from build123d import *

# Parameters (mm, degrees)
F0_W     = 42
F0_H     = 42
F1_DEPTH = 9.5
F3_DEPTH = 16.57
F4_W     = 42
F4_H     = 42
F5_DEPTH = 7.6
F7_DEPTH = 3
F8_R     = 2.5
F9_DEPTH = 24
F10_SIZE = 2
F11_R    = 1


with BuildPart() as f1:
    # F0 (on Top) → F1 (new body)
    with BuildSketch(Plane.XY):
        Rectangle(F0_W, F0_H)
    extrude(amount=F1_DEPTH)

    # F2 (on face) → F3 (join)
    with BuildSketch(Plane.XY.offset(9.5)):
        with BuildLine():
            Line((-16, -21), (16, -21))
            ThreePointArc((16, -21), (19.5355339059, -19.5355339059), (21, -16))
            Line((21, -16), (21, 16))
            ThreePointArc((21, 16), (19.5355339059, 19.5355339059), (16, 21))
            Line((16, 21), (-16, 21))
            ThreePointArc((-16, 21), (-19.5355339059, 19.5355339059), (-21, 16))
            Line((-21, 16), (-21, -16))
            ThreePointArc((-21, -16), (-19.5355339059, -19.5355339059), (-16, -21))
        make_face()
    extrude(amount=F3_DEPTH)

    # F4 (on face) → F5 (join)
    with BuildSketch(Plane.XY.offset(26.07)):
        Rectangle(F4_W, F4_H)
    extrude(amount=F5_DEPTH)

    # F6 (on face) → F7 (cut)
    with BuildSketch(Plane.XY.offset(33.67)):
        with BuildLine():
            Line((15.5, -14), (15.5, -15.5))
            Line((15.5, -15.5), (14, -15.5))
            ThreePointArc((14, -15.5), (15.5, -17), (17, -15.5))
            ThreePointArc((17, -15.5), (16.5606601718, -14.4393398282), (15.5, -14))
        make_face()
        with BuildLine():
            Line((14, -15.5), (15.5, -15.5))
            Line((15.5, -15.5), (15.5, -14))
            ThreePointArc((15.5, -14), (14.4393398282, -14.4393398282), (14, -15.5))
        make_face()
        with BuildLine():
            Line((15.5, 14), (15.5, 15.5))
            Line((15.5, 15.5), (14, 15.5))
            ThreePointArc((14, 15.5), (14.4393398282, 14.4393398282), (15.5, 14))
        make_face()
        with BuildLine():
            Line((14, 15.5), (15.5, 15.5))
            Line((15.5, 15.5), (15.5, 14))
            ThreePointArc((15.5, 14), (16.5606601718, 14.4393398282), (17, 15.5))
            ThreePointArc((17, 15.5), (15.5, 17), (14, 15.5))
        make_face()
        with BuildLine():
            Line((-14, -15.5), (-15.5, -15.5))
            Line((-15.5, -15.5), (-15.5, -14))
            ThreePointArc((-15.5, -14), (-16.5606601718, -16.5606601718), (-14, -15.5))
        make_face()
        with BuildLine():
            Line((-15.5, -14), (-15.5, -15.5))
            Line((-15.5, -15.5), (-14, -15.5))
            ThreePointArc((-14, -15.5), (-14.4393398282, -14.4393398282), (-15.5, -14))
        make_face()
        with BuildLine():
            Line((-15.5, 15.5), (-14, 15.5))
            ThreePointArc((-14, 15.5), (-16.5606601718, 16.5606601718), (-15.5, 14))
            Line((-15.5, 14), (-15.5, 15.5))
        make_face()
        with BuildLine():
            ThreePointArc((-15.5, 14), (-14.4393398282, 14.4393398282), (-14, 15.5))
            Line((-14, 15.5), (-15.5, 15.5))
            Line((-15.5, 15.5), (-15.5, 14))
        make_face()
    extrude(amount=-F7_DEPTH, mode=Mode.SUBTRACT)

    # F8 (on face) → F9 (join)
    with BuildSketch(Plane.XY.offset(33.67)):
        Circle(F8_R)
    extrude(amount=F9_DEPTH)

    # F10
    f10_edges = [f1.edges().sort_by_distance(p)[0] for p in [
        (21, 21, 29.87),
        (21, 21, 4.75),
        (-21, 21, 29.87),
        (-21, 21, 4.75),
        (-21, -21, 29.87),
        (-21, -21, 4.75),
        (21, -21, 4.75),
        (21, -21, 29.87),
    ]]
    chamfer(f10_edges, length=F10_SIZE)

    # F11
    f11_edges = [f1.edges().sort_by_distance(p)[0] for p in [
        (0, 21, 33.67),
        (-20, 20, 33.67),
        (-21, 0, 33.67),
        (-20, -20, 33.67),
        (0, -21, 33.67),
        (20, -20, 33.67),
        (21, 0, 33.67),
        (20, 20, 33.67),
        (0, 21, 0),
        (21, 0, 0),
        (20, 20, 0),
        (-21, 0, 0),
        (-20, 20, 0),
        (0, -21, 0),
        (20, -20, 0),
        (-20, -20, 0),
    ]]
    fillet(f11_edges, radius=F11_R)


solid = f1.part
The model under review builds one solid part; all positions refer to its coordinate system, in mm. A direction names the side the tool comes from. Coordinates: 2 decimals unless noted, no trailing zeros. Loops run counter-clockwise (first coordinate to the right, second up) from the corner with the lowest first, then second, coordinate; pieces in that order, holes last. Notation, with made-up numbers: (50, 9.25) -> (93, 9.25) arc R26 cw to (93, 35.25) -> close; hole circle Ø9 at (8.25, 89). An arc over 180 degrees is marked (long way). Use a Markdown table: item, result. Add a question column.
1. Add section A-A on x = 0. Write out the cut boundary in (y, z).
2. To check wall thickness, follow line 1 (X direction, y = -15.5, z = 32.55); line 2 (X direction, y = -15, z = 32). State the ranges of each line that lie inside material, in increasing order.
3. Add section C-C on z = 51.5. Write out the cut boundary in (x, y).
4. Clearance check with flat-ended pins moving along their axes: pin 1 Ø5.5 at (x, y) = (-19, -19.5) entering from +Z; pin 2 Ø0.9 at (x, y) = (-15.5, 15.5) entering from +Z; pin 3 Ø2 at (y, z) = (-1, 40.5) entering from +X. State where each tip first meets the part, or that it passes through.
5. Add section B-B on y = -7.5. Write out the cut boundary in (x, z), plus the area to 3 significant figures.
6. Draft analysis for pull direction Y (two halves, no side actions). For faces 5 (the face through (-20, 20, 5)), 6 (the face through (15, 16, 30.67)), 7 (the face through (-20, -19, 18)), state which applies: pulls with the +Y half, pulls with the -Y half, needs draft (parallel to the pull), parting line crosses it, or undercut.
7. Machinability: for faces 1 (the face through (19.6, 19.8, 9.5)), 2 (the face through (-16, -15, 30.67)), 3 (the face through (-19, 20, 18)), 4 (the face through (-19.8, -19.6, 26.07)), which of the approach directions +Z, -Z, +X, -X, +Y, -Y give a long, thin tool a straight path to every point of the face, cutting with its end or side? Answer none if there is none.
Returned:
| question | item | result |
|---|---|---|
| 1 | outline | (-21, 1) arc R1 ccw to (-20, 0) -> (20, 0) arc R1 ccw to (21, 1) -> (21, 32.67) arc R1 ccw to (20, 33.67) -> (2.5, 33.67) -> (2.5, 57.67) -> (-2.5, 57.67) -> (-2.5, 33.67) -> (-20, 33.67) arc R1 ccw to (-21, 32.67) -> close |
| 2 | line 1 | x = -21 to -17, -14 to 14, 17 to 21 |
| 2 | line 2 | x = -21 to -16.91, -14.09 to 14.09, 16.91 to 21 |
| 3 | outline | circle Ø5 at (0, 0) |
| 4 | pin 1 | stops at z = 33.67 |
| 4 | pin 2 | stops at z = 30.67 |
| 4 | pin 3 | stops at x = 2.5 |
| 5 | outline | (-21, 1) arc R1 ccw to (-20, 0) -> (20, 0) arc R1 ccw to (21, 1) -> (21, 32.67) arc R1 ccw to (20, 33.67) -> (-20, 33.67) arc R1 ccw to (-21, 32.67) -> close |
| 5 | area | 1,410 mm² |
| 6 | face 5 | pulls with the +Y half |
| 6 | face 6 | undercut |
| 6 | face 7 | pulls with the -Y half |
| 7 | face 1 | +X, +Y |
| 7 | face 2 | +Z |
| 7 | face 3 | -X, +Y |
| 7 | face 4 | -X, -Y |
